from build123d import *

# Parameters (mm, degrees)
BOSS_EXTRUDE1_DEPTH = 12.5
BOSS_EXTRUDE2_START = 12.5
BOSS_EXTRUDE2_DEPTH = 3
FILLET2_R           = 2
SHELL1_T            = -3
BOSS_EXTRUDE5_START = -20
SKETCH11_W          = 3
SKETCH11_H          = 2
BOSS_EXTRUDE5_DEPTH = 40
SKETCH12_W          = 6
SKETCH12_H          = 38
BOSS_EXTRUDE6_DEPTH = 3.5
SKETCH16_R          = 0.85
CUT_EXTRUDE5_DEPTH  = 4
CUT_EXTRUDE6_REACH  = 64.494
SKETCH17_R          = 1.75
SKETCH18_R          = 1.98
CUT_EXTRUDE7_DEPTH  = 1
CUT_EXTRUDE8_REACH  = 89.501
SKETCH19_W          = 20
SKETCH19_H          = 5
EXTRUDE_THIN1_START = 25
EXTRUDE_THIN1_DEPTH = 8
CUT_EXTRUDE9_START  = -12.5
SKETCH21_R          = 0.85
CUT_EXTRUDE9_DEPTH  = 4
CUT_EXTRUDE10_REACH = 64.494
SKETCH22_R          = 0.5
CUT_EXTRUDE12_REACH = 89.501
SKETCH23_R          = 2.5
CUT_EXTRUDE13_START = -6
SKETCH24_R          = 2.5
CUT_EXTRUDE13_DEPTH = 6
SKETCH25_R          = 8
SKETCH25_R_2        = 6
BOSS_EXTRUDE7_DEPTH = 2


with BuildPart() as part:
    # Sketch1 → Boss-Extrude1 (new, symmetric)
    with BuildSketch(Plane(origin=(0, 0, 0), x_dir=(1, 0, 0), z_dir=(0, 1, 0))):
        Polygon((-35.5, 23), (-23, 35.5), (23, 35.5), (35.5, 23), (35.5, -23), (23, -35.5), (-23, -35.5), (-35.5, -23), align=None)
    extrude(amount=BOSS_EXTRUDE1_DEPTH, both=True)

    # Sketch2 → Boss-Extrude2 (add)
    with BuildSketch(Plane(origin=(0, 0, 0), x_dir=(1, 0, 0), z_dir=(0, 1, 0)).offset(BOSS_EXTRUDE2_START)):
        with BuildLine():
            Line((-30.5, -40.5), (30.5, -40.5))
            ThreePointArc((30.5, -40.5), (37.571067812, -37.571067812), (40.5, -30.5))
            Line((40.5, -30.5), (40.5, 30.5))
            ThreePointArc((40.5, 30.5), (37.571067812, 37.571067812), (30.5, 40.5))
            Line((30.5, 40.5), (-30.5, 40.5))
            ThreePointArc((-30.5, 40.5), (-37.571067812, 37.571067812), (-40.5, 30.5))
            Line((-40.5, 30.5), (-40.5, -30.5))
            ThreePointArc((-40.5, -30.5), (-37.571067812, -37.571067812), (-30.5, -40.5))
        make_face()
    extrude(amount=BOSS_EXTRUDE2_DEPTH)

    # Fillet2
    fillet2_edges = [part.edges().sort_by_distance(p)[0] for p in [
        (0, 15.5, 40.5),
        (40.5, 15.5, 0),
        (0, 15.5, -40.5),
        (-40.5, 15.5, 0),
        (-37.571067812, 15.5, 37.571067812),
        (37.571067812, 15.5, 37.571067812),
        (37.571067812, 15.5, -37.571067812),
        (-37.571067812, 15.5, -37.571067812),
    ]]
    fillet(fillet2_edges, radius=FILLET2_R)

    # Shell1
    shell1_openings = [part.faces().sort_by_distance(p)[0] for p in [
        (0, -12.5, 0),
    ]]
    offset(amount=SHELL1_T, openings=shell1_openings, kind=Kind.INTERSECTION)

    # Sketch11 → Boss-Extrude5 (add)
    with BuildSketch(Plane(origin=(0, 0, 0), x_dir=(0, 0, -1), z_dir=(1, 0, 0)).offset(BOSS_EXTRUDE5_START)):
        with Locations((-31, 9.4)):
            Rectangle(SKETCH11_W, SKETCH11_H)
    extrude(amount=BOSS_EXTRUDE5_DEPTH)

    # Sketch12 → Boss-Extrude6 (add)
    with BuildSketch(Plane.XZ.offset(-12.5)):
        with Locations((-26, 6)):
            Rectangle(SKETCH12_W, SKETCH12_H)
        with Locations((26, 6)):
            Rectangle(SKETCH12_W, SKETCH12_H)
    extrude(amount=BOSS_EXTRUDE6_DEPTH)

    # Sketch16 → Cut-Extrude5 (cut)
    with BuildSketch(Plane.XZ.offset(-9)):
        with Locations(Location((26, 21, 0), (0, 0, 270))):
            Circle(SKETCH16_R)
        with Locations(Location((26, -9, 0), (0, 0, 270))):
            Circle(SKETCH16_R)
        with Locations(Location((-26, -9, 0), (0, 0, 90))):
            Circle(SKETCH16_R)
        with Locations(Location((-26, 21, 0), (0, 0, 90))):
            Circle(SKETCH16_R)
    extrude(amount=-CUT_EXTRUDE5_DEPTH, mode=Mode.SUBTRACT)

    # Sketch17 → Cut-Extrude6 (cut, up to next)
    with BuildSketch(Plane.XZ.offset(-12.5), mode=Mode.PRIVATE) as cut_extrude6_sk1:
        with Locations(Location((23.020139488, -21.613931872, 0), (0, 0, 270))):
            Circle(SKETCH17_R)
    cut_extrude6_tool1 = extrude(cut_extrude6_sk1.sketch, amount=-CUT_EXTRUDE6_REACH, mode=Mode.PRIVATE) & part.part
    add(cut_extrude6_tool1.solids().sort_by_distance((23.020139, 12.5, -21.613932))[0], mode=Mode.SUBTRACT)

    # Sketch18 → Cut-Extrude7 (cut)
    with BuildSketch(Plane.XZ.offset(-12.5)):
        with Locations(Location((23.020139488, -21.613931872, 0), (0, 0, 270))):
            Circle(SKETCH18_R)
    extrude(amount=-CUT_EXTRUDE7_DEPTH, mode=Mode.SUBTRACT)

    # Sketch19 → Cut-Extrude8 (cut, up to next)
    with BuildSketch(Plane.ZY.offset(35.5), mode=Mode.PRIVATE) as cut_extrude8_sk1:
        with Locations((0, 6)):
            Rectangle(SKETCH19_W, SKETCH19_H)
    cut_extrude8_tool1 = extrude(cut_extrude8_sk1.sketch, amount=-CUT_EXTRUDE8_REACH, mode=Mode.PRIVATE) & part.part
    add(cut_extrude8_tool1.solids().sort_by_distance((-35.5, 6, 0))[0], mode=Mode.SUBTRACT)

    # Sketch20 → Extrude-Thin1 (add)
    with BuildSketch(Plane.XZ.offset(-12.5).offset(EXTRUDE_THIN1_START)):
        Polygon((-32.5, 21.757359313), (-32.5, -21.757359313), (-21.757359313, -32.5), (21.757359313, -32.5), (32.5, -21.757359313), (32.5, 21.757359313), (21.757359313, 32.5), (-21.757359313, 32.5), align=None)
        Polygon((-29.5, 20.514718626), (-29.5, -20.514718626), (-20.514718626, -29.5), (20.514718626, -29.5), (29.5, -20.514718626), (29.5, 20.514718626), (20.514718626, 29.5), (-20.514718626, 29.5), align=None, mode=Mode.SUBTRACT)
    extrude(amount=-EXTRUDE_THIN1_DEPTH)

    # Sketch21 → Cut-Extrude9 (cut)
    with BuildSketch(Plane(origin=(0, 0, 0), x_dir=(1, 0, 0), z_dir=(0, 1, 0)).offset(CUT_EXTRUDE9_START)):
        with Locations(Location((0, -32.5, 0), (0, 0, 270))):
            Circle(SKETCH21_R)
        with Locations(Location((0, 32.5, 0), (0, 0, 270))):
            Circle(SKETCH21_R)
    extrude(amount=CUT_EXTRUDE9_DEPTH, mode=Mode.SUBTRACT)

    # Sketch22 → Cut-Extrude10 (cut, up to next)
    with BuildSketch(Plane.XZ.offset(-12.5), mode=Mode.PRIVATE) as cut_extrude10_sk1:
        with Locations(Location((-17, -23, 0), (0, 0, 270))):
            Circle(SKETCH22_R)
    cut_extrude10_tool1 = extrude(cut_extrude10_sk1.sketch, amount=-CUT_EXTRUDE10_REACH, mode=Mode.PRIVATE) & part.part
    # Sketch22 → Cut-Extrude10 (cut, up to next)
    with BuildSketch(Plane.XZ.offset(-12.5), mode=Mode.PRIVATE) as cut_extrude10_sk2:
        with Locations(Location((-15, -23, 0), (0, 0, 270))):
            Circle(SKETCH22_R)
    cut_extrude10_tool2 = extrude(cut_extrude10_sk2.sketch, amount=-CUT_EXTRUDE10_REACH, mode=Mode.PRIVATE) & part.part
    # Sketch22 → Cut-Extrude10 (cut, up to next)
    with BuildSketch(Plane.XZ.offset(-12.5), mode=Mode.PRIVATE) as cut_extrude10_sk3:
        with Locations(Location((-13, -23, 0), (0, 0, 270))):
            Circle(SKETCH22_R)
    cut_extrude10_tool3 = extrude(cut_extrude10_sk3.sketch, amount=-CUT_EXTRUDE10_REACH, mode=Mode.PRIVATE) & part.part
    # Sketch22 → Cut-Extrude10 (cut, up to next)
    with BuildSketch(Plane.XZ.offset(-12.5), mode=Mode.PRIVATE) as cut_extrude10_sk4:
        with Locations(Location((-15, -21, 0), (0, 0, 270))):
            Circle(SKETCH22_R)
    cut_extrude10_tool4 = extrude(cut_extrude10_sk4.sketch, amount=-CUT_EXTRUDE10_REACH, mode=Mode.PRIVATE) & part.part
    # Sketch22 → Cut-Extrude10 (cut, up to next)
    with BuildSketch(Plane.XZ.offset(-12.5), mode=Mode.PRIVATE) as cut_extrude10_sk5:
        with Locations(Location((-17, -21, 0), (0, 0, 270))):
            Circle(SKETCH22_R)
    cut_extrude10_tool5 = extrude(cut_extrude10_sk5.sketch, amount=-CUT_EXTRUDE10_REACH, mode=Mode.PRIVATE) & part.part
    # Sketch22 → Cut-Extrude10 (cut, up to next)
    with BuildSketch(Plane.XZ.offset(-12.5), mode=Mode.PRIVATE) as cut_extrude10_sk6:
        with Locations(Location((-13, -21, 0), (0, 0, 270))):
            Circle(SKETCH22_R)
    cut_extrude10_tool6 = extrude(cut_extrude10_sk6.sketch, amount=-CUT_EXTRUDE10_REACH, mode=Mode.PRIVATE) & part.part
    # Sketch22 → Cut-Extrude10 (cut, up to next)
    with BuildSketch(Plane.XZ.offset(-12.5), mode=Mode.PRIVATE) as cut_extrude10_sk7:
        with Locations(Location((-13, -19, 0), (0, 0, 90))):
            Circle(SKETCH22_R)
    cut_extrude10_tool7 = extrude(cut_extrude10_sk7.sketch, amount=-CUT_EXTRUDE10_REACH, mode=Mode.PRIVATE) & part.part
    # Sketch22 → Cut-Extrude10 (cut, up to next)
    with BuildSketch(Plane.XZ.offset(-12.5), mode=Mode.PRIVATE) as cut_extrude10_sk8:
        with Locations(Location((-15, -19, 0), (0, 0, 90))):
            Circle(SKETCH22_R)
    cut_extrude10_tool8 = extrude(cut_extrude10_sk8.sketch, amount=-CUT_EXTRUDE10_REACH, mode=Mode.PRIVATE) & part.part
    # Sketch22 → Cut-Extrude10 (cut, up to next)
    with BuildSketch(Plane.XZ.offset(-12.5), mode=Mode.PRIVATE) as cut_extrude10_sk9:
        with Locations(Location((-17, -19, 0), (0, 0, 90))):
            Circle(SKETCH22_R)
    cut_extrude10_tool9 = extrude(cut_extrude10_sk9.sketch, amount=-CUT_EXTRUDE10_REACH, mode=Mode.PRIVATE) & part.part
    add(cut_extrude10_tool1.solids().sort_by_distance((-17, 12.5, -23))[0], mode=Mode.SUBTRACT)
    add(cut_extrude10_tool2.solids().sort_by_distance((-15, 12.5, -23))[0], mode=Mode.SUBTRACT)
    add(cut_extrude10_tool3.solids().sort_by_distance((-13, 12.5, -23))[0], mode=Mode.SUBTRACT)
    add(cut_extrude10_tool4.solids().sort_by_distance((-15, 12.5, -21))[0], mode=Mode.SUBTRACT)
    add(cut_extrude10_tool5.solids().sort_by_distance((-17, 12.5, -21))[0], mode=Mode.SUBTRACT)
    add(cut_extrude10_tool6.solids().sort_by_distance((-13, 12.5, -21))[0], mode=Mode.SUBTRACT)
    add(cut_extrude10_tool7.solids().sort_by_distance((-13, 12.5, -19))[0], mode=Mode.SUBTRACT)
    add(cut_extrude10_tool8.solids().sort_by_distance((-15, 12.5, -19))[0], mode=Mode.SUBTRACT)
    add(cut_extrude10_tool9.solids().sort_by_distance((-17, 12.5, -19))[0], mode=Mode.SUBTRACT)

    # Sketch23 → Cut-Extrude12 (cut, up to next)
    with BuildSketch(Plane(origin=(0, 0, -35.5), x_dir=(-1, 0, 0), z_dir=(0, 0, -1)), mode=Mode.PRIVATE) as cut_extrude12_sk1:
        with Locations((0, 6)):
            Circle(SKETCH23_R)
    cut_extrude12_tool1 = extrude(cut_extrude12_sk1.sketch, amount=-CUT_EXTRUDE12_REACH, mode=Mode.PRIVATE) & part.part
    add(cut_extrude12_tool1.solids().sort_by_distance((0, 6, -35.5))[0], mode=Mode.SUBTRACT)

    # Sketch24 → Cut-Extrude13 (cut)
    with BuildSketch(Plane.XY.offset(35.5).offset(CUT_EXTRUDE13_START)):
        with Locations(Location((0, 6, 0), (0, 0, 180))):
            Circle(SKETCH24_R)
    extrude(amount=CUT_EXTRUDE13_DEPTH, mode=Mode.SUBTRACT)

    # Sketch25 → Boss-Extrude7 (add)
    with BuildSketch(Plane.XZ.offset(-12.5)):
        with Locations(Location((-15, -21, 0), (0, 0, 90))):
            Circle(SKETCH25_R)
        with Locations(Location((-15, -21, 0), (0, 0, 270))):
            Circle(SKETCH25_R_2, mode=Mode.SUBTRACT)
    extrude(amount=BOSS_EXTRUDE7_DEPTH)


solid = part.part
Part model, mm, in its own coordinate system. A direction names the side the tool comes from. Coordinates: 2 decimals unless noted, no trailing zeros. Write each loop counter-clockwise with the first axis right and the second up, starting at its lowest first coordinate (ties: lowest second). Pieces come first, ordered by that corner, then holes. Notation, with made-up numbers: (-33.75, 76) - (8.25, 76) arc R23 cw to (8.25, 87) - close; hole circle Ø9 at (50.5, 31.25). An arc over 180 degrees is marked (long way). Put each result on its own line as item: value.
1. Band-saw the part on A-A (y = 11.5). Give the number of separate pieces and of enclosed holes in the cut face, then the cut area to 3 significant figures.
Final values:
separate pieces: 4
enclosed holes: 6
area: 1,270 mm²
2. 3-axis set-ups, long thin cutter, end or side, ignore diameter. For faces 4 (the flat face through (29.2, 0.2, -29.3)), 5 (the flat face through (20, 9, 31)), 6 (the flat face through (-21, 10.5, -23)): which of +Z, -Z, +X, -X, +Y, -Y reach the whole face in a straight line?
Final values:
face 4: -Z, +X, -Y
face 5: none
face 6: -Y
3. Flat gauge pins, fed straight in: pin 1 Ø8.5 at (y, z) = (5.5, -7) entering from +X; pin 2 Ø10 at (x, y) = (11.5, 11) entering from +Z; pin 3 Ø1 at (y, z) = (0.5, -17.5) entering from -X; pin 4 Ø2.5 at (x, z) = (26, 21) entering from -Y. Where does each tip first touch, or does it go through?
Final values:
pin 1: stops at x = 35.5
pin 2: stops at z = 40.5
pin 3: stops at x = -35.5
pin 4: stops at y = 9
4. Two-plate mould, pull along Z, no slides. Class faces 1 (the cylindrical face through (0.33, 8.48, -34.02)), 2 (the flat face through (25.07, -8.556, 24.944)), 3 (the cylindrical face through (-37.49, 12.99, -37.65)): +Z half, -Z half, draft (parallel to the pull), parting line (faces both ways), or undercut.
Final values:
face 1: draft
face 2: undercut
face 3: -Z half
5. Band-saw the part on C-C (z = -11.5). Write the cut outline in (x, y), then the cut area to 3 significant figures.
Final values:
outline: (-40.5, 12.5) - (-35.5, 12.5) - (-35.5, -12.5) - (-29.5, -12.5) - (-29.5, -4.5) - (-32.5, -4.5) - (-32.5, 12.5) - (-29, 12.5) - (-29, 9) - (-23, 9) - (-23, 12.5) - (23, 12.5) - (23, 9) - (29, 9) - (29, 12.5) - (32.5, 12.5) - (32.5, -4.5) - (29.5, -4.5) - (29.5, -12.5) - (35.5, -12.5) - (35.5, 12.5) - (40.5, 12.5) - (40.5, 13.5) arc R2 ccw to (38.5, 15.5) - (-38.5, 15.5) arc R2 ccw to (-40.5, 13.5) - close
area: 481 mm²
6. Band-saw the part on B-B (y = 4.5). Write the cut outline in (x, z).
Final values:
outline: (-35.5, -23) - (-23, -35.5) - (-2, -35.5) - (-2, -32.5) - (-21.76, -32.5) - (-32.5, -21.76) - (-32.5, -10) - (-35.5, -10) - close; (-35.5, 10) - (-32.5, 10) - (-32.5, 21.76) - (-21.76, 32.5) - (-2, 32.5) - (-2, 35.5) - (-23, 35.5) - (-35.5, 23) - close; (2, -35.5) - (23, -35.5) - (35.5, -23) - (35.5, 23) - (23, 35.5) - (2, 35.5) - (2, 32.5) - (21.76, 32.5) - (32.5, 21.76) - (32.5, -21.76) - (21.76, -32.5) - (2, -32.5) - close
7. Band-saw the part on D-D (y = -9.5). Write the cut outline in (x, z), then the cut area to 3 significant figures.
Final values:
outline: (-35.5, -23) - (-23, -35.5) - (23, -35.5) - (35.5, -23) - (35.5, 23) - (23, 35.5) - (-23, 35.5) - (-35.5, 23) - close; hole (-29.5, -20.51) - (-20.51, -29.5) - (20.51, -29.5) - (29.5, -20.51) - (29.5, 20.51) - (20.51, 29.5) - (-20.51, 29.5) - (-29.5, 20.51) - close; hole circle Ø1.7 at (0, -32.5); hole circle Ø1.7 at (0, 32.5)
area: 1,400 mm²
8. Probe line 1 along X through (y, z) = (11.9, 21); line 2 along X through (y, z) = (-8, -6); line 3 along X through (y, z) = (13.75, -23). List the from-to ranges inside material, lowest first. Write a range as [from, to].
Final values:
line 1: x = [-35.5, -32.5], [-29, -26.85], [-25.15, -23], [23, 25.15], [26.85, 29], [32.5, 35.5]
line 2: x = [-35.5, -29.5], [29.5, 35.5]
line 3: x = [-40.48, -17.5], [-16.5, -15.5], [-14.5, -13.5], [-12.5, 21.95], [24.09, 40.48]
